Study the drawing (mm; zero at the part's minimum x, y, z) and answer. A direction names the side the tool comes from. Coordinates: 2 decimals unless noted, no trailing zeros. Order: outer loops, then holes, each group sorted by start corner. A loop starts at its lowest first (then second) coordinate and runs counter-clockwise, first axis right, second up. Notation, with made-up numbers: M 51.25,-4 L 75.25,-4 A34 cw 75.25,34 Z; hole C -20,56.5 d5. An arc over 180 degrees is marked long. One line per item, written item: value. Start each with the question number.
Q1. The part is cut by section A-A on z = 138. Give the vertices of the cut face in (x, y).
Q2. For the marked faces 5 and 6, determine the directions among +Z, -Z, +X, -X, +Y, -Y from which every point of the face is accessible in a straight line to the end or side of a thin tool.
Q3. Straight lines are drawn through the part: line 1 along X through (y, z) = (41, 236.5); line 2 along Y through (x, z) = (143.5, 81); line 3 along Z through (x, y) = (43, 6.5). For each, find the intervals that lie inside material, in ascending order. Write a range as [from, to].
Q4. The part is cut by section C-C on x = 17. Give the vertices of the cut face in (y, z), then the cut area to 3 significant figures.
Q5. Each of these flat-tipped pins is pushed along its axis until it touches: pin 1 Ø1 at (y, z) = (64, 150) entering from -X; pin 2 Ø10 at (y, z) = (64, 82.5) entering from -X; pin 3 Ø5 at (x, y) = (42.5, 23.5) entering from +Z; pin 4 Ø10 at (x, y) = (32, 51.5) entering from +Z. Where does it stop, or does it pass through?
Q6. The part is cut by section D-D on x = 75. Give the vertices of the cut face in (y, z), then the cut area to 3 significant figures.
Q7. Determine the mould class of the marked faces 1, 2, 3 and 4 for opening direction X: pulls with the +X half, pulls with the -X half, needs draft (parallel to the pull), parting line crosses it, or undercut.
Q8. The part is cut by section B-B on y = 45.5. Give the vertices of the cut face in (x, z), then the cut area to 3 significant figures.
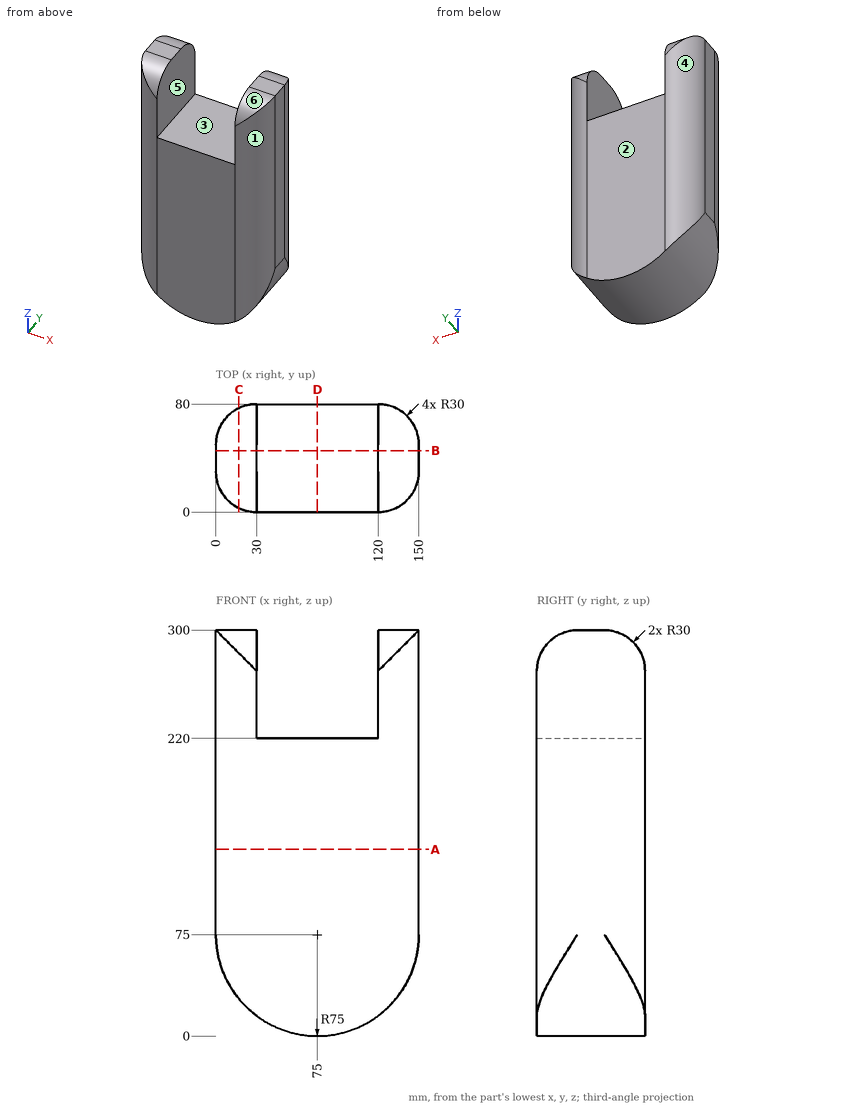
Output:
1. outline: M 0,30 A30 ccw 30,0 L 120,0 A30 ccw 150,30 L 150,50 A30 ccw 120,80 L 30,80 A30 ccw 0,50 Z
2. face 5: +Z, +Y, -Y
2. face 6: +Z, +X, -X, -Y
3. line 1: x = [0, 30], [120, 150]
3. line 2: y = [11.35, 68.65]
3. line 3: z = [7.17, 220]
4. outline: M 2.96,27.45 L 77.04,27.45 L 77.04,283 A30 ccw 50,300 L 30,300 A30 ccw 2.96,283 Z
4. area: 19,900 mm^2
5. pin 1: stops at x = 3.21
5. pin 2: stops at x = 1.38
5. pin 3: stops at z = 220
5. pin 4: stops at z = 300
6. outline: M 0,0 L 80,0 L 80,220 L 0,220 Z
6. area: 17,600 mm^2
7. face 1: pulls with the +X half
7. face 2: needs draft
7. face 3: undercut
7. face 4: pulls with the -X half
8. outline: M 0,75 A75 ccw 150,75 L 150,300 L 120,300 L 120,220 L 30,220 L 30,300 L 0,300 Z
8. area: 35,400 mm^2
